from build123d import *

# Parameters (mm, degrees)
SKETCH1_R                                      = 1.25
SHAPE_DEPTH                                    = 1
CSK_FOR_M2_FLAT_HEAD_MACHINE_SCREW1_AT_2_COUNT = 2
CSK_FOR_M2_FLAT_HEAD_MACHINE_SCREW1_AT_2_PITCH = 76.001699467
CSK_FOR_M2_FLAT_HEAD_MACHINE_SCREW1_AT_3_COUNT = 2
CSK_FOR_M2_FLAT_HEAD_MACHINE_SCREW1_AT_3_PITCH = 99.656702343
CSK_FOR_M2_FLAT_HEAD_MACHINE_SCREW1_AT_4_COUNT = 2
CSK_FOR_M2_FLAT_HEAD_MACHINE_SCREW1_AT_4_PITCH = 59.36
CSK_FOR_M2_FLAT_HEAD_MACHINE_SCREW1_AT_5_COUNT = 2
CSK_FOR_M2_FLAT_HEAD_MACHINE_SCREW1_AT_5_PITCH = 32.187410971
CSK_FOR_M2_FLAT_HEAD_MACHINE_SCREW1_AT_6_COUNT = 2
CSK_FOR_M2_FLAT_HEAD_MACHINE_SCREW1_AT_6_PITCH = 53.357546763


with BuildPart() as part:
    # Sketch1 → Shape (new body)
    with BuildSketch(Plane.XY):
        with BuildLine():
            Line((10.2, -38.3), (10.2, 38.3))
            Line((10.2, 38.3), (3.632299547, 38.3))
            ThreePointArc((3.632299547, 38.3), (3.220869448, 34.680909279), (0, 32.98))
            Line((0, 32.98), (-72.252025159, 32.98))
            Line((-72.252025159, 32.98), (-72.252025159, 25.630795063))
            ThreePointArc((-72.252025159, 25.630795063), (-69.552025159, 21.92), (-72.252025159, 18.209204937))
            Line((-72.252025159, 18.209204937), (-72.252025159, 16.789136368))
            ThreePointArc((-72.252025159, 16.789136368), (-59.422025159, 0), (-72.252025159, -16.789136368))
            Line((-72.252025159, -16.789136368), (-72.252025159, -18.209204937))
            ThreePointArc((-72.252025159, -18.209204937), (-69.552025159, -21.92), (-72.252025159, -25.630795063))
            Line((-72.252025159, -25.630795063), (-72.252025159, -32.98))
            Line((-72.252025159, -32.98), (0, -32.98))
            ThreePointArc((0, -32.98), (3.220869448, -34.680909279), (3.632299547, -38.3))
            Line((3.632299547, -38.3), (10.2, -38.3))
        make_face()
        with Locations((-68.952025159, 29.68)):
            Circle(SKETCH1_R, mode=Mode.SUBTRACT)
        with Locations((6.863249831, 35)):
            Circle(SKETCH1_R, mode=Mode.SUBTRACT)
        with Locations((6.863249831, -35)):
            Circle(SKETCH1_R, mode=Mode.SUBTRACT)
        with Locations((-68.952025159, -29.68)):
            Circle(SKETCH1_R, mode=Mode.SUBTRACT)
        with Locations((-56.497025159, 0)):
            Circle(SKETCH1_R, mode=Mode.SUBTRACT)
        with Locations((-24.61101258, 0)):
            Circle(SKETCH1_R, mode=Mode.SUBTRACT)
    extrude(amount=SHAPE_DEPTH)

    # Sketch3 → CSK for M2 Flat Head Machine Screw1 (revolve, cut)
    with BuildSketch(Plane(origin=(-68.952025159, 29.68, 1), x_dir=(0, -1, 0), z_dir=(1, 0, 0))):
        Polygon((0, 0), (0, 1), (1, 1), (1, 1.1), (2, 0.1), (2, 0), align=None)
    csk_for_m2_flat_head_machine_screw1 = revolve(axis=Axis((-68.952025159, 29.68, 7.35), (0, 0, -1)), mode=Mode.SUBTRACT)

    # CSK for M2 Flat Head Machine Screw1 at 2: CSK for M2 Flat Head Machine Screw1 ×2
    with Locations(*[Vector(0.997547101, 0.069998435, 0) * (i * CSK_FOR_M2_FLAT_HEAD_MACHINE_SCREW1_AT_2_PITCH) for i in range(1, CSK_FOR_M2_FLAT_HEAD_MACHINE_SCREW1_AT_2_COUNT)]):
        add(csk_for_m2_flat_head_machine_screw1, mode=Mode.SUBTRACT)

    # CSK for M2 Flat Head Machine Screw1 at 3: CSK for M2 Flat Head Machine Screw1 ×2
    with Locations(*[Vector(0.760764436, -0.649028098, 0) * (i * CSK_FOR_M2_FLAT_HEAD_MACHINE_SCREW1_AT_3_PITCH) for i in range(1, CSK_FOR_M2_FLAT_HEAD_MACHINE_SCREW1_AT_3_COUNT)]):
        add(csk_for_m2_flat_head_machine_screw1, mode=Mode.SUBTRACT)

    # CSK for M2 Flat Head Machine Screw1 at 4: CSK for M2 Flat Head Machine Screw1 ×2
    with Locations(*[(0, -i * CSK_FOR_M2_FLAT_HEAD_MACHINE_SCREW1_AT_4_PITCH, 0) for i in range(1, CSK_FOR_M2_FLAT_HEAD_MACHINE_SCREW1_AT_4_COUNT)]):
        add(csk_for_m2_flat_head_machine_screw1, mode=Mode.SUBTRACT)

    # CSK for M2 Flat Head Machine Screw1 at 5: CSK for M2 Flat Head Machine Screw1 ×2
    with Locations(*[Vector(0.386952527, -0.922099638, 0) * (i * CSK_FOR_M2_FLAT_HEAD_MACHINE_SCREW1_AT_5_PITCH) for i in range(1, CSK_FOR_M2_FLAT_HEAD_MACHINE_SCREW1_AT_5_COUNT)]):
        add(csk_for_m2_flat_head_machine_screw1, mode=Mode.SUBTRACT)

    # CSK for M2 Flat Head Machine Screw1 at 6: CSK for M2 Flat Head Machine Screw1 ×2
    with Locations(*[Vector(0.831016703, -0.556247463, 0) * (i * CSK_FOR_M2_FLAT_HEAD_MACHINE_SCREW1_AT_6_PITCH) for i in range(1, CSK_FOR_M2_FLAT_HEAD_MACHINE_SCREW1_AT_6_COUNT)]):
        add(csk_for_m2_flat_head_machine_screw1, mode=Mode.SUBTRACT)


solid = part.part
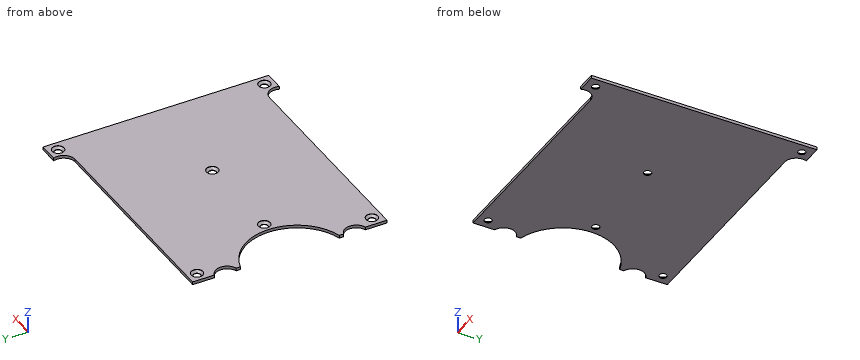
Geometry: final body of the model. Coordinates: model frame, mm. Coordinates: 2 decimals unless noted, no trailing zeros. Write each loop counter-clockwise with the first axis right and the second up, starting at its lowest first coordinate (ties: lowest second). Pieces come first, ordered by that corner, then holes. Notation, with made-up numbers: (-23, 53.5) - (-10, 53.5) arc R19 cw to (-10, 87.5) - close; hole circle Ø8 at (74.25, -39.75). An arc over 180 degrees is marked (long way). Return JSON: item names as keys, results as strings.
Item 1: Section query C-C (z = 0.5). Output: boundary loops of the cut face in (x, y).
Completed:
{"outline": "(-72.25, -32.98) - (0, -32.98) arc R3.9 cw to (3.63, -38.3) - (10.2, -38.3) - (10.2, 38.3) - (3.63, 38.3) arc R3.9 cw to (0, 32.98) - (-72.25, 32.98) - (-72.25, 25.63) arc R3.9 cw to (-72.25, 18.21) - (-72.25, 16.79) arc R17.4 cw to (-72.25, -16.79) - (-72.25, -18.21) arc R3.9 cw to (-72.25, -25.63) - close; hole circle Ø3.2 at (-68.95, -29.68); hole circle Ø3.2 at (-68.95, 29.68); hole circle Ø3.2 at (-56.5, 0); hole circle Ø3.2 at (-24.61, 0); hole circle Ø3.2 at (6.86, -35); hole circle Ø3.2 at (6.86, 35)"}
Item 2: Section query A-A (y = 0). Output: boundary loops of the cut face in (x, z), and give its area (3 significant figures).
Completed:
{"outline": "(-59.42, 0) - (-57.75, 0) - (-57.75, 0.15) - (-58.5, 0.9) - (-58.5, 1) - (-59.42, 1) - close; (-55.25, 0) - (-25.86, 0) - (-25.86, 0.15) - (-26.61, 0.9) - (-26.61, 1) - (-54.5, 1) - (-54.5, 0.9) - (-55.25, 0.15) - close; (-23.36, 0) - (10.2, 0) - (10.2, 1) - (-22.61, 1) - (-22.61, 0.9) - (-23.36, 0.15) - close", "area": "63.2 mm2"}
Item 3: Section query D-D (x = -42.5). Output: boundary loops of the cut face in (y, z).
Completed:
{"outline": "(-32.98, 0) - (32.98, 0) - (32.98, 1) - (-32.98, 1) - close"}
Item 4: Pin query (flat end, axial travel): pin 1 Ø3 at (x, y) = (-68.95, -29.68) entering from +Z. Return the tip coordinate at first contact, or that it passes through.
Completed:
{"pin 1": "stops at z = 0.4"}
Item 5: Section query B-B (y = 29.68). Output: boundary loops of the cut face in (x, z), and give its area (3 significant figures).
Completed:
{"outline": "(-72.25, 0) - (-70.2, 0) - (-70.2, 0.15) - (-70.95, 0.9) - (-70.95, 1) - (-72.25, 1) - close; (-67.7, 0) - (10.2, 0) - (10.2, 1) - (-66.95, 1) - (-66.95, 0.9) - (-67.7, 0.15) - close", "area": "79.2 mm2"}
Item 6: Line query: L1, parallel to X at y = -0.5, z = 0.55; L2, parallel to Y at x = 7, z = 0.25; L3, parallel to Y at x = -29, z = 0.8. Output: solid intervals per line, ascending.
Completed:
{"L1": "x = -59.43 to -58.07, -54.92 to -26.18, -23.04 to 10.2", "L2": "y = -38.3 to -36.34, -33.66 to 33.66, 36.34 to 38.3", "L3": "y = -32.98 to 32.98"}
